```python
from build123d import *

# Parameters (mm, degrees)
F0_R     = 3.75
F1_DEPTH = 5
F2_DEPTH = 10
F3_DEPTH = 5


with BuildPart() as f1:
    # F0 (on Top) → F1 (new body)
    with BuildSketch(Plane.XY):
        with BuildLine():
            Line((35, 12.5), (0, 12.5))
            add(Edge.make_bspline(
                [(0, 12.5), (9.166667, 12.5), (18.333333, 0), (27.5, -12.5)],
                knots=[37.165172, 37.165172, 37.165172, 37.165172, 74.330344, 74.330344, 74.330344, 74.330344], degree=3))
            Line((27.5, -12.5), (35, -12.5))
            Line((35, -12.5), (35, 12.5))
        make_face()
        with BuildLine():
            Line((0, 12.5), (-35, 12.5))
            Line((-35, 12.5), (-35, -12.5))
            Line((-35, -12.5), (-27.5, -12.5))
            add(Edge.make_bspline(
                [(-27.5, -12.5), (-18.333333, 0), (-9.166667, 12.5), (0, 12.5)],
                knots=[0, 0, 0, 0, 37.165172, 37.165172, 37.165172, 37.165172], degree=3))
        make_face()
        with BuildLine():
            add(Edge.make_bspline(
                [(0, 12.5), (9.166667, 12.5), (18.333333, 0), (27.5, -12.5)],
                knots=[37.165172, 37.165172, 37.165172, 37.165172, 74.330344, 74.330344, 74.330344, 74.330344], degree=3))
            add(Edge.make_bspline(
                [(-27.5, -12.5), (-18.333333, 0), (-9.166667, 12.5), (0, 12.5)],
                knots=[0, 0, 0, 0, 37.165172, 37.165172, 37.165172, 37.165172], degree=3))
            Line((-27.5, -12.5), (-5, -12.5))
            Line((-5, -12.5), (5, -12.5))
            Line((5, -12.5), (27.5, -12.5))
        make_face()
        with Locations((0, 2.5)):
            Circle(F0_R, mode=Mode.SUBTRACT)
        Polygon((5, -12.5), (-5, -12.5), (-5, -17.5), (-12.5, -17.5), (-12.5, -22.5), (-5, -22.5), (-5, -27.5), (0, -27.5), (5, -27.5), (5, -22.5), (12.5, -22.5), (12.5, -17.5), (5, -17.5), align=None)
    extrude(amount=F1_DEPTH)

    # F0 (on Top) → F2 (join)
    with BuildSketch(Plane.XY):
        with BuildLine():
            add(Edge.make_bspline(
                [(0, 12.5), (9.166667, 12.5), (18.333333, 0), (27.5, -12.5)],
                knots=[37.165172, 37.165172, 37.165172, 37.165172, 74.330344, 74.330344, 74.330344, 74.330344], degree=3))
            add(Edge.make_bspline(
                [(-27.5, -12.5), (-18.333333, 0), (-9.166667, 12.5), (0, 12.5)],
                knots=[0, 0, 0, 0, 37.165172, 37.165172, 37.165172, 37.165172], degree=3))
            Line((-27.5, -12.5), (-5, -12.5))
            Line((-5, -12.5), (5, -12.5))
            Line((5, -12.5), (27.5, -12.5))
        make_face()
        with Locations((0, 2.5)):
            Circle(F0_R, mode=Mode.SUBTRACT)
        Polygon((5, -12.5), (-5, -12.5), (-5, -17.5), (-12.5, -17.5), (-12.5, -22.5), (-5, -22.5), (-5, -27.5), (0, -27.5), (5, -27.5), (5, -22.5), (12.5, -22.5), (12.5, -17.5), (5, -17.5), align=None)
    extrude(amount=-F2_DEPTH)

    # F0 (on Top) → F3 (join)
    with BuildSketch(Plane.XY):
        with Locations((0, 2.5)):
            Circle(F0_R)
    extrude(amount=F3_DEPTH)


solid = f1.part
```
Read the model definition and answer for the solid it produces. Units are mm, in the model's axes. A direction names the side the tool comes from. Give positions to 0.01 mm unless a question says otherwise; leave off trailing zeros. Loops run counter-clockwise (first coordinate to the right, second up) from the corner with the lowest first, then second, coordinate; pieces in that order, holes last.
Item 1: The part is cut by section A-A (z = 1.5). Write down the section's boundary in (x, y), and give its area (4 significant figures).
Item 2: The mould has two halves that part along Y. Classify faces 4 (the flat face through (-35, 0, 2)), 5 (the flat face through (-9, -22.5, -2)), 6 (the cylindrical face through (-0.488, 6.218, -4.93)): released by +Y, released by -Y, zero draft, split by the parting line, or undercut.
Item 3: For faces 1 (the flat face through (-5, -15, -2)), 2 (the flat face through (5, -15, -2)), 3 (the flat face through (-26, 3, 0)), determine the directions among +Z, -Z, +X, -X, +Y, -Y from which every point of the face is accessible in a straight line to the end or side of a thin tool.
Item 4: The part is cut by section C-C (y = -16). Write down the section's boundary in (x, z), and give its area (3 significant figures).
Item 5: Each of these flat-tipped pins is pushed along its axis until it touches: pin 1 Ø20 at (x, y) = (-19.5, 3) entering from -Z; pin 2 Ø1.5 at (x, y) = (-21, -2.5) entering from -Z; pin 3 Ø2.5 at (y, z) = (-19, -4) entering from +X; pin 4 Ø1.5 at (y, z) = (-15, -6) entering from -X. Where does it stop, or does it pass through?
Item 6: Find the intervals of material crossed by line 1 along Y through (x, z) = (0, -2); line 2 along X through (y, z) = (-24, -1.75); line 3 along X through (y, z) = (5.5, -2.25), in increasing order.
Item 7: The part is cut by section B-B (x = -29). Write down the section's boundary in (y, z).
Taken from the geometry:
1. outline: (-35, -12.5) - (-5, -12.5) - (-5, -17.5) - (-12.5, -17.5) - (-12.5, -22.5) - (-5, -22.5) - (-5, -27.5) - (5, -27.5) - (5, -22.5) - (12.5, -22.5) - (12.5, -17.5) - (5, -17.5) - (5, -12.5) - (35, -12.5) - (35, 12.5) - (-35, 12.5) - close
1. area: 1,975 mm2
2. face 4: zero draft
2. face 5: released by -Y
2. face 6: undercut
3. face 1: +Z, -Z, -X
3. face 2: +Z, -Z, +X
3. face 3: -Z, -X, +Y
4. outline: (-5, -10) - (5, -10) - (5, 5) - (-5, 5) - close
4. area: 150 mm2
5. pin 1: stops at z = -10
5. pin 2: stops at z = 0
5. pin 3: stops at x = 12.5
5. pin 4: stops at x = -5
6. line 1: y = -27.5 to -1.25, 6.25 to 12.5
6. line 2: x = -5 to 5
6. line 3: x = -12.94 to -2.25, 2.25 to 12.94
7. outline: (-12.5, 0) - (12.5, 0) - (12.5, 5) - (-12.5, 5) - close
